Model file for the job. Use its own axes, mm. A direction names the side the tool comes from. Round coordinates to 2 decimals unless told otherwise and drop trailing zeros. Loops run counter-clockwise (first coordinate to the right, second up) from the corner with the lowest first, then second, coordinate; pieces in that order, holes last. Notation, with made-up numbers: (52, 19.25) -> (104, 19.25) arc R8 cw to (104, 27.25) -> close; hole circle Ø9 at (2, -38.75). An arc over 180 degrees is marked (long way). Use a Markdown table: item, result.
from build123d import *

# Parameters (mm, degrees)
SKETCH1_R           = 24.6126
BOSS_EXTRUDE1_DEPTH = 9.525
BOSS_EXTRUDE2_START = 9.525
SKETCH2_R           = 12.7
BOSS_EXTRUDE2_DEPTH = 35.7124
SKETCH3_R           = 8.7122
BOSS_EXTRUDE4_DEPTH = 4.826
SKETCH4_R           = 2.7686
CUT_EXTRUDE2_DEPTH  = 58.078739617
FILLET1_R           = 0.381
FILLET2_R           = 2.3876
CHAMFER1_SIZE       = 0.762
CHAMFER2_SIZE       = 1.524


with BuildPart() as part:
    # Sketch1 → Boss-Extrude1 (new body)
    with BuildSketch(Plane.YZ):
        with Locations(Location((0, 0, 0), (0, 0, 270))):
            Circle(SKETCH1_R)
    extrude(amount=BOSS_EXTRUDE1_DEPTH)

    # Sketch2 → Boss-Extrude2 (add)
    with BuildSketch(Plane.YZ.offset(BOSS_EXTRUDE2_START)):
        with Locations(Location((0, 0, 0), (0, 0, 270))):
            Circle(SKETCH2_R)
    extrude(amount=BOSS_EXTRUDE2_DEPTH)

    # Sketch3 → Boss-Extrude4 (add)
    with BuildSketch(Plane.YZ):
        with Locations(Location((0, 0, 0), (0, 0, 270))):
            Circle(SKETCH3_R)
    extrude(amount=-BOSS_EXTRUDE4_DEPTH)

    # Sketch4 → Cut-Extrude2 (cut, through all)
    with BuildSketch(Plane.YZ):
        with Locations((24.6126, 44.45)):
            Circle(SKETCH4_R)
        with Locations((44.45, 24.6126)):
            Circle(SKETCH4_R)
        with Locations((24.6126, 4.7752)):
            Circle(SKETCH4_R)
        with Locations((4.7752, 24.6126)):
            Circle(SKETCH4_R)
    extrude(amount=CUT_EXTRUDE2_DEPTH, mode=Mode.SUBTRACT)

    # Fillet1
    fillet1_edges = [part.edges().sort_by_distance(p)[0] for p in [
        (0, 0, 8.7122),
    ]]
    fillet(fillet1_edges, radius=FILLET1_R)

    # Fillet2
    fillet2_edges = [part.edges().sort_by_distance(p)[0] for p in [
        (9.525, 0, 12.7),
    ]]
    fillet(fillet2_edges, radius=FILLET2_R)

    # Chamfer1
    chamfer1_edges = [part.edges().sort_by_distance(p)[0] for p in [
        (0, 17.403736363, 17.403736363),
        (0, -17.403736363, -17.403736363),
        (9.525, 17.403736363, 17.403736363),
        (9.525, -17.403736363, -17.403736363),
    ]]
    chamfer(chamfer1_edges, length=CHAMFER1_SIZE)

    # Chamfer2
    chamfer2_edges = [part.edges().sort_by_distance(p)[0] for p in [
        (45.2374, 0, 12.7),
    ]]
    chamfer(chamfer2_edges, length=CHAMFER2_SIZE)


solid = part.part
Q1. Band-saw the part on A-A, the plane z = 0. Give the cut face in (x, y) (3 decimals), plus the area to 3 significant figures.
Results list:
| item | result |
|---|---|
| outline | (-4.826, -8.712) -> (-0.381, -8.712) arc R0.381 cw to (0, -9.093) -> (0, -23.851) -> (0.762, -24.613) -> (8.763, -24.613) -> (9.525, -23.851) -> (9.525, -15.088) arc R2.388 cw to (11.913, -12.7) -> (43.713, -12.7) -> (45.237, -11.176) -> (45.237, 11.176) -> (43.713, 12.7) -> (11.913, 12.7) arc R2.388 cw to (9.525, 15.088) -> (9.525, 23.851) -> (8.763, 24.613) -> (0.762, 24.613) -> (0, 23.851) -> (0, 9.093) arc R0.381 cw to (-0.381, 8.712) -> (-4.826, 8.712) -> close |
| area | 1,460 mm² |
Q2. Band-saw the part on C-C, the plane x = 39. Give the cut face in (y, z).
Results list:
| item | result |
|---|---|
| outline | circle Ø25.4 at (0, 0) |
Q3. Pull direction Y, two halves, no side cores. Call faces 1 (the face through (4.696, 4.197, 21.905)), 2 (the face through (9.39, -16.37, -17.53)), 3 (the face through (4.706, 17.521, 17.285)): released by +Y, released by -Y, zero draft, split by the parting line, or undercut.
Results list:
| item | result |
|---|---|
| face 1 | undercut |
| face 2 | split by the parting line |
| face 3 | released by +Y |
Q4. Drill centre lines: L1, parallel to X at y = -19, z = 11 (3 decimals); L2, parallel to Z at x = 3, y = -18; L3, parallel to Y at x = 30, z = 9. Where is each one in solid material? Low to high. Write a range as from..to.
Results list:
| item | result |
|---|---|
| L1 | x = 0..9.525 |
| L2 | z = -16.79..16.79 |
| L3 | y = -8.96..8.96 |
Q5. Flat gauge pins, fed straight in: pin 1 (2 mm diameter, centred on x = 37, y = -7, fed in from +Z); pin 2 (1 mm diameter, centred on x = 25.5, z = -11, fed in from +Y); pin 3 (12 mm diameter, centred on x = 33.5, z = 8.5, fed in from -Y). Where does each tip first touch, or does it go through?
Results list:
| item | result |
|---|---|
| pin 1 | stops at z = 11.19 |
| pin 2 | stops at y = 7.14 |
| pin 3 | stops at y = -12.45 |
Q6. Tool access for faces 4 (the face through (4.696, 21.885, 4.299)), 5 (the face through (0, -10, 0)), 6 (the face through (27.6, -7.7, 10.1)): list every direction of +Z, -Z, +X, -X, +Y, -Y with a clear straight run to the whole face (end or side of a thin tool).
Results list:
| item | result |
|---|---|
| face 4 | +X, -X, +Y |
| face 5 | -X |
| face 6 | +X |
